Work out the finished part from the listing and answer in its coordinate system (mm). Face numbers are marked on the shaded views. Coordinates: 2 decimals unless noted, no trailing zeros. Loops run counter-clockwise (first coordinate to the right, second up) from the corner with the lowest first, then second, coordinate; pieces in that order, holes last. Notation, with made-up numbers: M -25,62.25 L 20,62.25 A32 ccw 20,92.25 Z; hole C 87,44 d10. An arc over 180 degrees is marked long. Write each question's results on one line, items separated by ' | '.
```python
from build123d import *

# Parameters (mm, degrees)
SKETCH1_R                                      = 15.24
BOSS_EXTRUDE1_DEPTH                            = 6.35
CBORE_FOR_2_SOCKET_HEAD_CAP_SCREW1_D           = 2.2606
CBORE_FOR_2_SOCKET_HEAD_CAP_SCREW1_CBORE_D     = 4.7625
CBORE_FOR_2_SOCKET_HEAD_CAP_SCREW1_CBORE_DEPTH = 2.1844
CIRPATTERN1_COUNT                              = 3
CIRPATTERN2_COUNT                              = 3
CIRPATTERN3_COUNT                              = 3
SKETCH16_R                                     = 5.08
CUT_EXTRUDE1_DEPTH                             = 6.35


with BuildPart() as part:
    # Sketch1 → Boss-Extrude1 (new body)
    with BuildSketch(Plane(origin=(0, 0, 0), x_dir=(1, 0, 0), z_dir=(0, 1, 0))):
        with Locations(Location((0, 0, 0), (0, 0, 270))):
            Circle(SKETCH1_R)
    extrude(amount=BOSS_EXTRUDE1_DEPTH)

    # CBORE for #2 Socket Head Cap Screw1 (through all)
    with Locations(Plane(origin=(0, 6.35, 0), x_dir=(1, 0, 0), z_dir=(0, 1, 0))):
        with Locations((7.363810019, -7.363810019)):
            cbore_for_2_socket_head_cap_screw1 = CounterBoreHole(CBORE_FOR_2_SOCKET_HEAD_CAP_SCREW1_D / 2, CBORE_FOR_2_SOCKET_HEAD_CAP_SCREW1_CBORE_D / 2, CBORE_FOR_2_SOCKET_HEAD_CAP_SCREW1_CBORE_DEPTH)

    # CirPattern1: CBORE for #2 Socket Head Cap Screw1 ×3 about axis
    cirpattern1_axis = Axis((0, 0, 0), (0, 1, 0))
    for i in range(1, CIRPATTERN1_COUNT):
        add(cbore_for_2_socket_head_cap_screw1.rotate(cirpattern1_axis, i * 360 / CIRPATTERN1_COUNT), mode=Mode.SUBTRACT)

    # Sketch10 → Tap Drill for #2-56 Tap2 (revolve, cut)
    with BuildSketch(Plane(origin=(7.977586831, 6.35, -6.693990167), x_dir=(0, 0, 1), z_dir=(1, 0, 0))):
        Polygon((0, 0), (0, 4.59816509), (0.889, 4.064), (0.889, 0), align=None)
    tap_drill_for_2_56_tap2 = revolve(axis=Axis((7.977586831, 12.7, -6.693990167), (0, -1, 0)), mode=Mode.SUBTRACT)

    # CirPattern2: Tap Drill for #2-56 Tap2 ×3 about axis
    cirpattern2_axis = Axis((0, 0, 0), (0, 1, 0))
    for i in range(1, CIRPATTERN2_COUNT):
        add(tap_drill_for_2_56_tap2.rotate(cirpattern2_axis, i * 360 / CIRPATTERN2_COUNT), mode=Mode.SUBTRACT)

    # Sketch15 → Tap Drill for #2-56 Tap1 (revolve, cut)
    with BuildSketch(Plane(origin=(-7.57363795, 3.105629072, 13.224885943), x_dir=(0.8677746681735182, 0, 0.49695787072581954), z_dir=(0, 1, 0))):
        Polygon((0, 0), (0, 7.095959572), (0.889, 6.35), (0.889, 0), align=None)
    tap_drill_for_2_56_tap1 = revolve(axis=Axis((-10.729320429, 3.105629072, 18.735255086), (0.4969578707258196, 0, -0.8677746681735182)), mode=Mode.SUBTRACT)

    # CirPattern3: Tap Drill for #2-56 Tap1 ×3 about axis
    cirpattern3_axis = Axis((0, 6.35, 0), (0, -1, 0))
    for i in range(1, CIRPATTERN3_COUNT):
        add(tap_drill_for_2_56_tap1.rotate(cirpattern3_axis, i * 360 / CIRPATTERN3_COUNT), mode=Mode.SUBTRACT)

    # Sketch16 → Cut-Extrude1 (cut)
    with BuildSketch(Plane(origin=(0, 6.35, 0), x_dir=(1, 0, 0), z_dir=(0, 1, 0))):
        with Locations(Location((0, 0, 0), (0, 0, 270))):
            Circle(SKETCH16_R)
    extrude(amount=-CUT_EXTRUDE1_DEPTH, mode=Mode.SUBTRACT)


solid = part.part
```
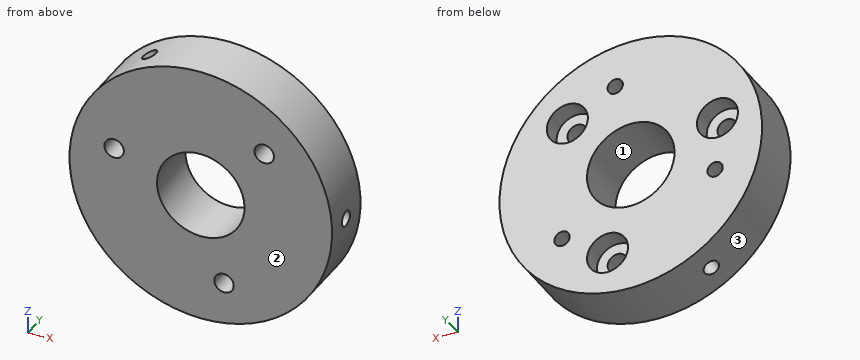
1) Find section A-A, the plane y = 5. Give the vertices of the cut face in (x, z) (1 decimal), and give its area (3 significant figures).
Check result:
outline: C 0,0 d30.5; hole C -10.1,2.7 d4.8; hole C -9.8,-3.6 d1.8; hole C 0,0 d10.2; hole C 2.7,-10.1 d4.8; hole C 1.8,10.3 d1.8; hole C 7.4,7.4 d4.8; hole C 8,-6.7 d1.8 | area: 588 mm^2
2) Find section B-B, the plane y = 1.25. Give the vertices of the cut face in (x, z).
Check result:
outline: C 0,0 d30.48; hole C -10.06,2.7 d2.26; hole C 0,0 d10.16; hole C 2.7,-10.06 d2.26; hole C 7.36,7.36 d2.26
3) Straight lines are drawn through the part: probe 1 along X at (y, z) = (6, -3); probe 2 along Z at (x, y) = (7.5, 3.5); probe 3 along Z at (x, y) = (1, 2.5). For each, find the intervals that lie inside material, in ascending order. Write a range as [from, to].
Check result:
probe 1: [-14.94, -10.47], [-9.1, -4.1], [4.1, 14.94] | probe 2: [-13.27, -7.44], [-5.94, 6.24], [8.49, 13.27] | probe 3: [-15.21, -4.98], [4.98, 9.89], [10.63, 15.21]
4) Given pin 1 Ø3.5 at (x, z) = (2.7, -10.06) entering from +Y; pin 2 Ø6 at (x, z) = (0, 0) entering from +Y (3 decimals); pin 3 Ø2 at (x, y) = (-11, 4) entering from -Z; pin 4 Ø1.5 at (x, y) = (9.5, 5) entering from -Z, each flat-ended and moving along its own axis, determine where each tip first touches the part or whether it passes through.
Check result:
pin 1: y = 4.17 | pin 2: through | pin 3: z = -11.5 | pin 4: z = -12.48
5) For a pull along X with two mould halves and no side action, classify the marked faces 1, 2 and 3 as released by +X, released by -X, zero draft, split by the parting line, or undercut.
Check result:
face 1: undercut | face 2: zero draft | face 3: split by the parting line
